CAD build for the part. Positions are in the model's coordinates, mm. Coordinates: 2 decimals unless noted, no trailing zeros. Loops run counter-clockwise (first coordinate to the right, second up) from the corner with the lowest first, then second, coordinate; pieces in that order, holes last. Notation, with made-up numbers: (-13, 81) -> (34, 81) arc R7 cw to (34, 89) -> close; hole circle Ø10 at (-38.75, -9.5). An arc over 180 degrees is marked (long way). Return JSON: item names as keys, results as strings. Group by question number.
(1) Mould opens along X. For faces 1 (the face through (-0.53, 24.21, 1.57)), 2 (the face through (-3.083, -13.886, 1.565)), 3 (the face through (35.922, -75.759, 1.565)) say: pulls with the +X half, pulls with the -X half, needs draft (parallel to the pull), parting line crosses it, or undercut.
(2) Flat gauge pin, fed straight in: pin 1 Ø12 at (x, y) = (-34.5, -126) entering from -Z. Where does the tip first touch, or does it go through?
(3) Saw through at B-B on y = -104. Write the cut outline in (x, z) (3 decimals), then the cut area to 3 significant figures.
(4) Saw through at A-A on x = 0. Write the cut outline in (y, z) (3 decimals).
(5) Saw through at D-D on z = 1.65. Write the cut outline in (x, y).
(6) Saw through at C-C on x = -18.5. Write the cut outline in (y, z) (1 decimal), then the cut area to 3 significant figures.
(7) Probe L1, parallel to Y at x = 0, z = 2.15; L2, parallel to X at y = 0.5, z = 1.95; L3, parallel to Y at x = -3.5, z = 2.4. List the from-to ranges inside material, lowest first.
```python
from build123d import *

# Parameters (mm, degrees)
SKETCH1_R           = 14.224
BOSS_EXTRUDE1_DEPTH = 3.175
SKETCH2_R           = 32.004
CUT_EXTRUDE1_DEPTH  = 3.175


with BuildPart() as part:
    # Sketch1 → Boss-Extrude1 (new body)
    with BuildSketch(Plane.XY):
        with BuildLine():
            Line((47.961011706, -153.67), (-47.961011706, -153.67))
            Line((-47.961011706, -153.67), (-24.216066116, 0))
            ThreePointArc((-24.216066116, 0), (0, 24.216066116), (24.216066116, 0))
            Line((24.216066116, 0), (47.961011706, -153.67))
        make_face()
        Circle(SKETCH1_R, mode=Mode.SUBTRACT)
    extrude(amount=BOSS_EXTRUDE1_DEPTH)

    # Sketch2 → Cut-Extrude1 (cut)
    with BuildSketch(Plane.XY.offset(3.175)):
        with Locations((0, -112.056738627)):
            Circle(SKETCH2_R)
    extrude(amount=-CUT_EXTRUDE1_DEPTH, mode=Mode.SUBTRACT)


solid = part.part
```
Geometry results:
{
 "1": {"face 1": "parting line crosses it", "face 2": "undercut", "face 3": "pulls with the +X half"},
 "2": {"pin 1": "z = 0"},
 "3": {"outline": "(-40.286, 0) -> (-30.973, 0) -> (-30.973, 3.175) -> (-40.286, 3.175) -> close; (30.973, 0) -> (40.286, 0) -> (40.286, 3.175) -> (30.973, 3.175) -> close", "area": "59.1 mm²"},
 "4": {"outline": "(-153.67, 0) -> (-144.061, 0) -> (-144.061, 3.175) -> (-153.67, 3.175) -> close; (-80.053, 0) -> (-14.224, 0) -> (-14.224, 3.175) -> (-80.053, 3.175) -> close; (14.224, 0) -> (24.216, 0) -> (24.216, 3.175) -> (14.224, 3.175) -> close"},
 "5": {"outline": "(-47.96, -153.67) -> (47.96, -153.67) -> (24.22, 0) arc R24.22 ccw to (-24.22, 0) -> close; hole circle Ø64.01 at (0, -112.06); hole circle Ø28.45 at (0, 0)"},
 "6": {"outline": "(-153.7, 0) -> (-138.2, 0) -> (-138.2, 3.2) -> (-153.7, 3.2) -> close; (-85.9, 0) -> (15.6, 0) -> (15.6, 3.2) -> (-85.9, 3.2) -> close", "area": "372 mm²"},
 "7": {"L1": "-153.67 to -144.06, -80.05 to -14.22, 14.22 to 24.22", "L2": "-24.21 to -14.22, 14.22 to 24.21", "L3": "-153.67 to -143.87, -80.24 to -13.79, 13.79 to 23.96"}
}
